Verification items for the finished model (mm, model axes). A direction names the side the tool comes from. Give positions to 0.01 mm unless a question says otherwise; leave off trailing zeros. Order: outer loops, then holes, each group sorted by start corner. A loop starts at its lowest first (then second) coordinate and runs counter-clockwise, first axis right, second up. Notation, with made-up numbers: (-32.75, -14) - (-3.75, -14) arc R11 ccw to (-3.75, 4) - close; hole circle Ø6 at (56.25, 3). An arc over 180 degrees is marked (long way). Answer as a JSON object with one key per item and string values. Group by question number.
(1) Section check B-B (x = 66.5). Record the boundary of the cut face in (y, z), then the cut area to 3 significant figures.
(2) Mould release check, pull along X, two halves, no side actions. Record for faces 1 (the face through (-84.803, 0, 212)), 2 (the face through (93.677, 3.3, 9.9)), 3 (the face through (-2.1, -93.587, 406.6)): +X half, -X half, draft (parallel to the pull), parting line (faces both ways), or undercut.
(3) Access from +Z, -Z, +X, -X, +Y, -Y to the whole of each face (thin tool, end or side, straight path). Record for faces 4 (the face through (0, 84.803, 212)), 5 (the face through (-3.3, 93.677, 408.9)).
(4) Section check C-C (y = -67). Record the boundary of the cut face in (x, z), then the cut area to 3 significant figures.
(5) Depth check by flat-ended pin: pin 1 Ø5.5 at (x, z) = (0, 409) entering from -Y; pin 2 Ø12 at (x, z) = (0, 150) entering from -Y; pin 3 Ø2 at (x, z) = (-10, 278) entering from -Y. Enter the tip coordinate at first touch or a pass-through.
(6) Thickness scan on line 1 (Y direction, x = -3.5, z = 188); line 2 (X direction, y = 32.5, z = 81); line 3 (Y direction, x = -10, z = 166). Record the ranges inside material, lowest first.
(7) Section check A-A (z = 220.5). Record the boundary of the cut face in (x, y), then the cut area to 3 significant figures.
```python
from build123d import *
from build123d.topology import SkipClean

# Parameters (mm, degrees)
EXTRUDE_1_DEPTH          = 419
CUT_EXTRUDE_START        = -399
SKETCH_2_R               = 110
SKETCH_2_R_2             = 90
CUT_EXTRUDE_1_DEPTH      = 379
SKETCH_3_R               = 84
CUT_EXTRUDE_2_DEPTH      = 440.444628006
SKETCH_4_W               = 15.5
SKETCH_4_H               = 1
SKETCH_4_W_2             = 1
SKETCH_4_H_2             = 11.5
SKETCH_4_W_3             = 11.5
CUT_EXTRUDE_3_DEPTH      = 440.444628006
SKETCH_5_R               = 3
CUT_EXTRUDE_4_DEPTH      = 465.963674458
PATTERN_CIRCULAR_1_COUNT = 4


with BuildPart() as part:
    # 草图1 → 凸台-拉伸1 (new body)
    with BuildSketch(Plane.XY):
        with BuildLine():
            Line((-8.75, -89.573642887), (-8.75, -93.587458654))
            Line((-8.75, -93.587458654), (8.75, -93.587458654))
            Line((8.75, -93.587458654), (8.75, -89.573642887))
            ThreePointArc((8.75, -89.573642887), (63.993668164, -63.283571604), (89.66569857, -7.75))
            Line((89.66569857, -7.75), (93.676520759, -7.75))
            Line((93.676520759, -7.75), (93.676520759, 7.75))
            Line((93.676520759, 7.75), (89.66569857, 7.75))
            ThreePointArc((89.66569857, 7.75), (63.639610307, 63.639610307), (7.75, 89.66569857))
            Line((7.75, 89.66569857), (7.75, 93.676520759))
            Line((7.75, 93.676520759), (-7.75, 93.676520759))
            Line((-7.75, 93.676520759), (-7.75, 89.66569857))
            ThreePointArc((-7.75, 89.66569857), (-63.639610307, 63.639610307), (-89.66569857, 7.75))
            Line((-89.66569857, 7.75), (-93.676520759, 7.75))
            Line((-93.676520759, 7.75), (-93.676520759, -7.75))
            Line((-93.676520759, -7.75), (-89.66569857, -7.75))
            ThreePointArc((-89.66569857, -7.75), (-63.993668164, -63.283571604), (-8.75, -89.573642887))
        make_face()
    extrude(amount=EXTRUDE_1_DEPTH)

    # 草图2 → 切除-拉伸1 (cut)
    with SkipClean():  # the faces are left unmerged after this step: merging them gives an invalid solid
        with BuildSketch(Plane.XY.offset(419).offset(CUT_EXTRUDE_START)):
            Circle(SKETCH_2_R)
            with Locations(Location((0, 0, 0), (0, 0, 184.939921132))):
                Circle(SKETCH_2_R_2, mode=Mode.SUBTRACT)
        extrude(amount=CUT_EXTRUDE_1_DEPTH, mode=Mode.SUBTRACT)

    # 草图3 → 切除-拉伸2 (cut, through all)
    with SkipClean():  # the faces are left unmerged after this step: merging them gives an invalid solid
        with BuildSketch(Plane.XY.offset(419)):
            Circle(SKETCH_3_R)
        extrude(amount=-CUT_EXTRUDE_2_DEPTH, mode=Mode.SUBTRACT)

    # 草图4 → 切除-拉伸3 (cut, through all)
    with SkipClean():  # the faces are left unmerged after this step: merging them gives an invalid solid
        with BuildSketch(Plane.XY.offset(419)):
            with Locations((0, -84.141721049)):
                Rectangle(SKETCH_4_W, SKETCH_4_H)
            with Locations((-84.302968325, 0)):
                Rectangle(SKETCH_4_W_2, SKETCH_4_H_2)
            with Locations((0, 84.302968325)):
                Rectangle(SKETCH_4_W_3, SKETCH_4_H)
            with Locations((84.302968325, 0)):
                Rectangle(SKETCH_4_W_2, SKETCH_4_H_2)
        extrude(amount=-CUT_EXTRUDE_3_DEPTH, mode=Mode.SUBTRACT)

    # 草图5 → 切除-拉伸4 (cut, through all)
    with SkipClean():  # the faces are left unmerged after this step: merging them gives an invalid solid
        with BuildSketch(Plane(origin=(-84.802968325, 0, 0), x_dir=(0, 0, -1), z_dir=(1, 0, 0))):
            with Locations((-409, 0)):
                Circle(SKETCH_5_R)
            with Locations((-10, 0)):
                Circle(SKETCH_5_R)
        cut_extrude_4 = extrude(amount=-CUT_EXTRUDE_4_DEPTH, mode=Mode.SUBTRACT)

    # 阵列(圆周)1: 切除-拉伸4 ×4 about axis
    with SkipClean():  # the faces are left unmerged after this step: merging them gives an invalid solid
        pattern_circular_1_axis = Axis((0, 0, 1000), (0, 0, -1))
        for i in range(1, PATTERN_CIRCULAR_1_COUNT):
            add(cut_extrude_4.rotate(pattern_circular_1_axis, i * 360 / PATTERN_CIRCULAR_1_COUNT), mode=Mode.SUBTRACT)


solid = part.part
```
Solutions:
{
 "1": {"outline": "(-60.64, 0) - (-51.32, 0) - (-51.32, 419) - (-60.64, 419) - close; (51.32, 0) - (60.64, 0) - (60.64, 419) - (51.32, 419) - close", "area": "7,810 mm2"},
 "2": {"face 1": "undercut", "face 2": "+X half", "face 3": "draft"},
 "3": {"face 4": "+Z, -Z", "face 5": "+Z, -Z, +X, -X, +Y"},
 "4": {"outline": "(-60.09, 0) - (-50.67, 0) - (-50.67, 419) - (-60.09, 419) - close; (50.67, 0) - (60.09, 0) - (60.09, 419) - (50.67, 419) - close", "area": "7,900 mm2"},
 "5": {"pin 1": "stops at y = -84.8", "pin 2": "stops at y = -90", "pin 3": "stops at y = -89.55"},
 "6": {"line 1": "y = -89.93 to -84.64, 84.8 to 89.93", "line 2": "x = -83.93 to -77.46, 77.46 to 83.93", "line 3": "y = -89.44 to -83.4, 83.4 to 89.44"},
 "7": {"outline": "circle Ø180 at (0, 0); hole (-84.8, -5.75) - (-83.8, -5.75) arc R84 ccw to (-7.75, -83.64) - (-7.75, -84.64) - (7.75, -84.64) - (7.75, -83.64) arc R84 ccw to (83.8, -5.75) - (84.8, -5.75) - (84.8, 5.75) - (83.8, 5.75) arc R84 ccw to (5.75, 83.8) - (5.75, 84.8) - (-5.75, 84.8) - (-5.75, 83.8) arc R84 ccw to (-83.8, 5.75) - (-84.8, 5.75) - close", "area": "3,240 mm2"}
}
